Geometry: final body of the model. Coordinates: model frame, mm. Give positions to 0.01 mm unless a question says otherwise; leave off trailing zeros. Loops run counter-clockwise (first coordinate to the right, second up) from the corner with the lowest first, then second, coordinate; pieces in that order, holes last.
```python
from build123d import *

# Parameters (mm, degrees)
F0_W     = 304.8
F0_H     = 457.2
F1_DEPTH = 19.05
F2_R     = 5.08
F3_R     = 5.08
F4_W     = 304.8
F4_H     = 297.3566651344
F5_DEPTH = 19.05
F7_R     = 5.08
F8_R     = 5.08


with BuildPart() as f1:
    # F0 (on Front) → F1 (new body)
    with BuildSketch(Plane.XZ):
        with BuildLine():
            ThreePointArc((304.8, 457.2), (152.4, 609.6), (0, 457.2))
            Line((0, 457.2), (304.8, 457.2))
        make_face()
        with Locations((152.4, 228.6)):
            Rectangle(F0_W, F0_H)
        with BuildLine():
            Line((304.8, 0), (0, 0))
            ThreePointArc((0, 0), (152.4, -152.4), (304.8, 0))
        make_face()
    extrude(amount=F1_DEPTH)

    # F2
    f2_edges = [f1.edges().sort_by_distance(p)[0] for p in [
        (0, -19.05, 228.6),
        (152.4, -19.05, 609.6),
        (304.8, -19.05, 228.6),
        (152.4, -19.05, -152.4),
    ]]
    fillet(f2_edges, radius=F2_R)

    # F3
    f3_edges = [f1.edges().sort_by_distance(p)[0] for p in [
        (304.8, 0, 228.6),
        (152.4, 0, 609.6),
        (0, 0, 228.6),
        (152.4, 0, -152.4),
    ]]
    fillet(f3_edges, radius=F3_R)


with BuildPart() as f5:
    # F4 (on Front) → F5 (new body)
    with BuildSketch(Plane.XZ):
        with Locations((152.4, 148.6783325672)):
            Rectangle(F4_W, F4_H)
        with BuildLine():
            ThreePointArc((304.8, 297.3566651344), (152.4, 449.7566651344), (0, 297.3566651344))
            Line((0, 297.3566651344), (304.8, 297.3566651344))
        make_face()
        with BuildLine():
            Line((304.8, 0), (0, 0))
            ThreePointArc((0, 0), (152.4, -152.4), (304.8, 0))
        make_face()
    extrude(amount=F5_DEPTH)

    # F7
    f7_edges = [f5.edges().sort_by_distance(p)[0] for p in [
        (0, -19.05, 148.678333),
        (152.4, -19.05, 449.756665),
        (304.8, -19.05, 148.678333),
        (152.4, -19.05, -152.4),
    ]]
    fillet(f7_edges, radius=F7_R)

    # F8
    f8_edges = [f5.edges().sort_by_distance(p)[0] for p in [
        (304.8, 0, 148.678333),
        (152.4, 0, 449.756665),
        (0, 0, 148.678333),
        (152.4, 0, -152.4),
    ]]
    fillet(f8_edges, radius=F8_R)


solid = f5.part
```
Q1. Section query A-A, the plane y = -8.75. Return loops of the section in (x, z).
Q2. Pin query (flat end, axial travel): pin 1 Ø10 at (x, y) = (76.5, -8) entering from +Z; pin 2 Ø10 at (x, y) = (246.5, -3.5) entering from +Z; pin 3 Ø10 at (x, y) = (53, -7) entering from -Z. Return the tip coordinate at first contact, or that it passes through.
Q3. Material intervals for probe 1 along Z at (x, y) = (154, -8); probe 2 along X at (y, z) = (-17, 158); probe 3 along Z at (x, y) = (195.5, -11.5), sorted ascending.
Resolved:
1. outline: (0, 0) arc R152.4 ccw to (304.8, 0) - (304.8, 297.36) arc R152.4 ccw to (0, 297.36) - close
2. pin 1: stops at z = 432.26
2. pin 2: stops at z = 420.88
2. pin 3: stops at z = -119.64
3. probe 1: z = -152.39 to 449.75
3. probe 2: x = 1 to 303.8
3. probe 3: z = -146.18 to 443.54
